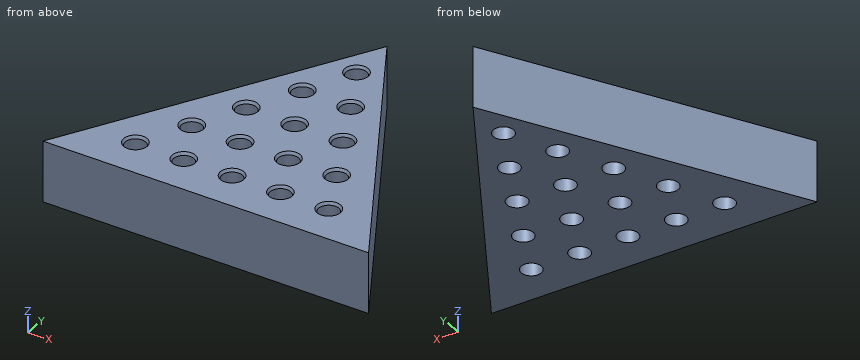
from build123d import *

# Parameters (mm, degrees)
F7_DEPTH = 19.05
F1_R     = 3.175
F2_R     = 3.175
F3_R     = 3.175
F4_R     = 3.175
F5_R     = 3.175
F8_DEPTH = 25.4
F9_SIZE2 = 0.879882
F9_SIZE  = 0.508


with BuildPart() as f7:
    # F6 (on face) → F7 (new body)
    with BuildSketch(Plane.XY):
        Polygon((-8.272192, 0), (94.380685, 0), (43.054246, 88.9), align=None)
    extrude(amount=F7_DEPTH)

    # F1 (on face) + F2 (on face) + F3 (on face) + F4 (on face) + F5 (on face) → F8 (cut)
    with BuildSketch(Plane.XY):
        with Locations((12.7, 12.7)):
            Circle(F1_R)
        with Locations((27.94, 12.7)):
            Circle(F1_R)
        with Locations((43.18, 12.7)):
            Circle(F1_R)
        with Locations((58.42, 12.7)):
            Circle(F1_R)
        with Locations((73.66, 12.7)):
            Circle(F1_R)
    with BuildSketch(Plane.XY):
        with Locations((20.669391, 27.935994)):
            Circle(F2_R)
        with Locations((35.909391, 27.935994)):
            Circle(F2_R)
        with Locations((51.149391, 27.935994)):
            Circle(F2_R)
        with Locations((66.389391, 27.935994)):
            Circle(F2_R)
    with BuildSketch(Plane.XY):
        with Locations((28.076159, 43.175994)):
            Circle(F3_R)
        with Locations((43.316159, 43.175994)):
            Circle(F3_R)
        with Locations((58.556159, 43.175994)):
            Circle(F3_R)
    with BuildSketch(Plane.XY):
        with Locations((35.941, 58.415994)):
            Circle(F4_R)
        with Locations((51.181, 58.415994)):
            Circle(F4_R)
    with BuildSketch(Plane.XY):
        with Locations((43.2308, 73.655994)):
            Circle(F5_R)
    extrude(amount=F8_DEPTH, mode=Mode.SUBTRACT)

    # F9
    f9_edges = [f7.edges().sort_by_distance(p)[0] for p in [
        (9.525, 12.7, 19.05),
        (24.765, 12.7, 19.05),
        (40.005, 12.7, 19.05),
        (55.245, 12.7, 19.05),
        (70.485, 12.7, 19.05),
        (63.214391, 27.935994, 19.05),
        (47.974391, 27.935994, 19.05),
        (32.734391, 27.935994, 19.05),
        (17.494391, 27.935994, 19.05),
        (24.901159, 43.175994, 19.05),
        (40.141159, 43.175994, 19.05),
        (55.381159, 43.175994, 19.05),
        (48.006, 58.415994, 19.05),
        (32.766, 58.415994, 19.05),
        (40.0558, 73.655994, 19.05),
    ]]
    chamfer(f9_edges, length=F9_SIZE, length2=F9_SIZE2)


solid = f7.part
Verification items for the finished model (mm, model axes). Round coordinates to 2 decimals unless told otherwise and drop trailing zeros. Loops run counter-clockwise (first coordinate to the right, second up) from the corner with the lowest first, then second, coordinate; pieces in that order, holes last. Notation, with made-up numbers: (16.5, 68) - (41.5, 68) arc R32 ccw to (41.5, 104) - close; hole circle Ø7 at (-37.5, 30). An arc over 180 degrees is marked (long way). Use a Markdown table: item, result. Add a question column.
1. Section check A-A, the plane x = 73.66. Record the boundary of the cut face in (y, z) (3 decimals), plus the area to 3 significant figures.
2. Gauge pin test, flat ends, axial feed: pin 1 (6 mm diameter, centred on y = 19, z = 11, fed in from +X); pin 2 (5 mm diameter, centred on x = 35.91, y = 27.94, fed in from +Z); pin 3 (1 mm diameter, centred on y = 19.5, z = 2, fed in from +X); pin 4 (8 mm diameter, centred on y = 57, z = 13, fed in from +X). Record the tip position at first contact, or that the pin passes through.
3. Thickness scan on probe 1 along X at (y, z) = (42, 17); probe 2 along X at (y, z) = (26.5, 13); probe 3 along Y at (x, z) = (43.5, 8). Record the ranges inside material, lowest first. Write a range as [from, to].
4. Section check B-B, the plane z = 10.25. Give the number of separate pieces and of enclosed holes in the cut face, plus the area to 3 significant figures.
Checks:
| question | item | result |
|---|---|---|
| 1 | outline | (0, 0) - (9.525, 0) - (9.525, 18.17) - (9.017, 19.05) - (0, 19.05) - close; (15.875, 0) - (35.889, 0) - (35.889, 19.05) - (16.383, 19.05) - (15.875, 18.17) - close |
| 1 | area | 562 mm^2 |
| 2 | pin 1 | stops at x = 85.14 |
| 2 | pin 2 | passes through |
| 2 | pin 3 | stops at x = 83.41 |
| 2 | pin 4 | stops at x = 63.78 |
| 3 | probe 1 | x = [15.98, 25.13], [31.03, 40.37], [46.27, 55.61], [61.51, 70.13] |
| 3 | probe 2 | x = [7.03, 17.84], [23.5, 33.08], [38.74, 48.32], [53.98, 63.56], [69.22, 79.08] |
| 3 | probe 3 | y = [0, 9.54], [15.86, 40.01], [46.35, 70.49], [76.82, 88.13] |
| 4 | separate pieces | 1 |
| 4 | enclosed holes | 15 |
| 4 | area | 4,090 mm^2 |
